Design review of the part built by this model. Coordinates are the model's own, in mm. Coordinates: 2 decimals unless noted, no trailing zeros. Loops run counter-clockwise (first coordinate to the right, second up) from the corner with the lowest first, then second, coordinate; pieces in that order, holes last. Notation, with made-up numbers: M 69.25,66.25 L 76.25,66.25 A29 cw 76.25,105.25 Z; hole C 71,45 d5. An arc over 180 degrees is marked long. Answer as a JSON object with one key per item and string values. Group by question number.
1. Consider section D-D (x = -34). State the section outline as (y, z) points, then the cut area to 3 significant figures.
2. Consider section C-C (x = -13). State the section outline as (y, z) points.
3. Consider section A-A (z = -15). State the section outline as (x, y) points, then the cut area to 3 significant figures.
4. Consider section B-B (y = 1.5). State the section outline as (x, z) points.
5. To check wall thickness, follow probe 1 along X at (y, z) = (1.35, -15); probe 2 along Z at (x, y) = (-13.5, 0.75). State the ranges of each line that lie inside material, in increasing order.
6. Insertion check: pin 1 (4 mm diameter, centred on x = -15, z = -15, fed in from +Y). The pin has a flat end and moves straight along its axis. Give the tip position at first contact, or say it passes through.
7. Draft analysis for pull direction Z (two halves, no side actions). For faces 1 (the flat face through (0, 1, -29)), 2 (the flat face through (-30, 1, 0)), 3 (the cylindrical face through (-14.577, 0.986, -18.222)), state which applies: +Z half, -Z half, draft (parallel to the pull), parting line (faces both ways), or undercut.
from build123d import *

# Parameters (mm, degrees)
EXTRUDE1_DEPTH                 = 2
F_6_5_6_5_DIAMETER_HOLE1_D     = 6.5
F_6_5_6_5_DIAMETER_HOLE1_DEPTH = 2


with BuildPart() as part:
    # Sketch1 → Extrude1 (new body)
    with BuildSketch(Plane(origin=(0, 0, 0), x_dir=(1, 0, 0), z_dir=(0, 1, 0))):
        Polygon((-40, 0), (-18.786796564, 0), (0, 18.786796564), (0, 40), align=None)
    extrude(amount=EXTRUDE1_DEPTH)

    # Ø6.5 (6.5) Diameter Hole1
    with Locations(Plane(origin=(0, 2, 0), x_dir=(1, 0, 0), z_dir=(0, 1, 0))):
        with Locations((-15, 15)):
            Hole(F_6_5_6_5_DIAMETER_HOLE1_D / 2, depth=F_6_5_6_5_DIAMETER_HOLE1_DEPTH)


solid = part.part
Findings below:
{
 "1": {"outline": "M 0,-6 L 2,-6 L 2,0 L 0,0 Z", "area": "12.0 mm^2"},
 "2": {"outline": "M 0,-27 L 2,-27 L 2,-17.56 L 0,-17.56 Z; M 0,-12.44 L 2,-12.44 L 2,-5.79 L 0,-5.79 Z"},
 "3": {"outline": "M -25,0 L -18.25,0 L -18.25,2 L -25,2 Z; M -11.75,0 L -3.79,0 L -3.79,2 L -11.75,2 Z", "area": "29.4 mm^2"},
 "4": {"outline": "M -40,0 L 0,-40 L 0,-18.79 L -18.79,0 Z; hole C -15,-15 d6.5"},
 "5": {"probe 1": "x = -25 to -18.25, -11.75 to -3.79", "probe 2": "z = -26.5 to -17.88, -12.12 to -5.29"},
 "6": {"pin 1": "passes through"},
 "7": {"face 1": "draft", "face 2": "+Z half", "face 3": "undercut"}
}
